Part print with two shaded views. Sizes in mm from the minimum x, y, z corner. A direction names the side the tool comes from. Round coordinates to 2 decimals unless told otherwise and drop trailing zeros. Order: outer loops, then holes, each group sorted by start corner. A loop starts at its lowest first (then second) coordinate and runs counter-clockwise, first axis right, second up. Notation, with made-up numbers: (27, 73.25) -> (44, 73.25) arc R32 cw to (44, 104.25) -> close; hole circle Ø3 at (-37.75, 48.5). An arc over 180 degrees is marked (long way). Use a Markdown table: item, result. Add a question column.
Item 1: 3-axis set-ups, long thin cutter, end or side, ignore diameter. For the marked faces 1 and 2: which of +Z, -Z, +X, -X, +Y, -Y reach the whole face in a straight line?
Item 2: Probe L1, parallel to Z at x = 8.75, y = 10; L2, parallel to Y at x = 6, z = 0.25; L3, parallel to X at y = 6.75, z = 0.25. List the from-to ranges inside material, lowest first.
Item 3: Slice it at D-D, the plane x = 8.25. Give the cut face in (y, z).
Item 4: Slice it at A-A, the plane x = 6. Give the cut face in (y, z), plus the area to 3 significant figures.
Item 5: Pin check, flat tips, straight feed: pin 1 (3.5 mm diameter, centred on x = 4, y = 7.5, fed in from +Z); pin 2 (0.5 mm diameter, centred on y = 12, z = 1.5, fed in from +X); pin 3 (2 mm diameter, centred on x = 5, y = 5, fed in from +Z); pin 4 (0.8 mm diameter, centred on y = 12, z = 1.5, fed in from -X). Stop position of each tip, or through.
Item 6: Slice it at B-B, the plane y = 6. Give the cut face in (x, z), plus the area to 3 significant figures.
Item 7: Slice it at C-C, the plane z = 0.35. Give the cut face in (x, y).
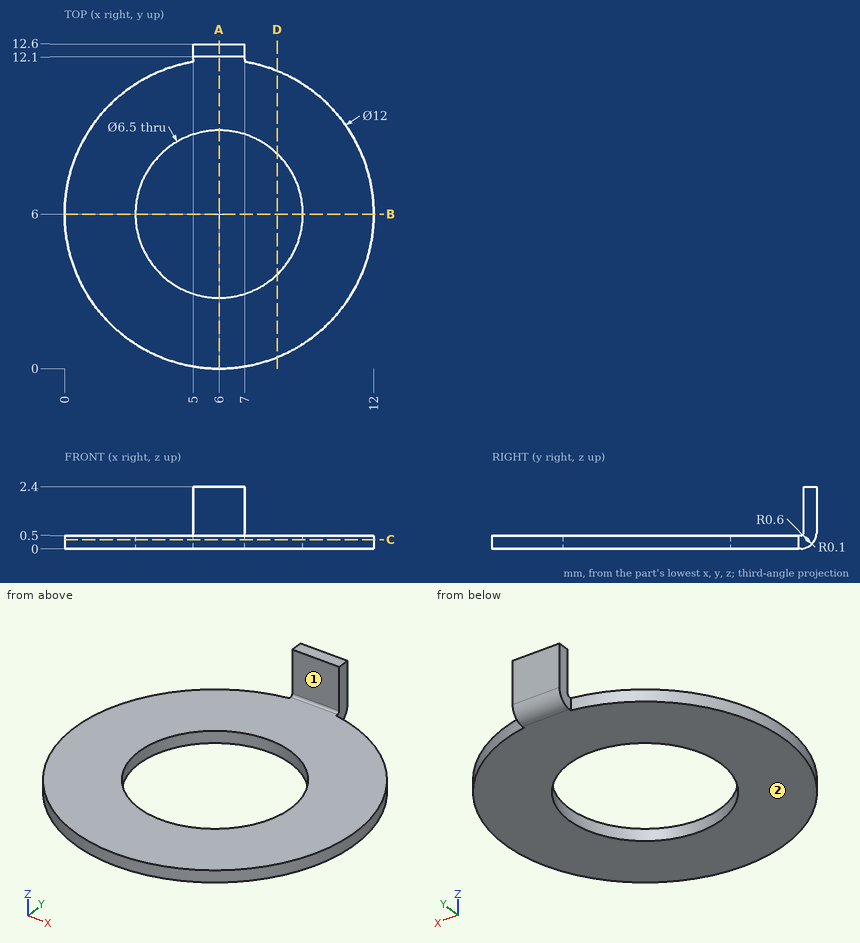
Check sheet entries:
| question | item | result |
|---|---|---|
| 1 | face 1 | +Z, +X, -X, -Y |
| 1 | face 2 | -Z, +X, -X, +Y, -Y |
| 2 | L1 | 0 to 0.5 |
| 2 | L2 | 0 to 2.75, 9.25 to 12.49 |
| 2 | L3 | 0.05 to 2.84, 9.16 to 11.95 |
| 3 | outline | (0.44, 0) -> (3.65, 0) -> (3.65, 0.5) -> (0.44, 0.5) -> close; (8.35, 0) -> (11.56, 0) -> (11.56, 0.5) -> (8.35, 0.5) -> close |
| 4 | outline | (0, 0) -> (2.75, 0) -> (2.75, 0.5) -> (0, 0.5) -> close; (9.25, 0) -> (12, 0) arc R0.6 ccw to (12.6, 0.6) -> (12.6, 2.4) -> (12.1, 2.4) -> (12.1, 0.6) arc R0.1 cw to (12, 0.5) -> (9.25, 0.5) -> close |
| 4 | area | 3.92 mm2 |
| 5 | pin 1 | z = 0.5 |
| 5 | pin 2 | x = 7 |
| 5 | pin 3 | through |
| 5 | pin 4 | x = 5 |
| 6 | outline | (0, 0) -> (2.75, 0) -> (2.75, 0.5) -> (0, 0.5) -> close; (9.25, 0) -> (12, 0) -> (12, 0.5) -> (9.25, 0.5) -> close |
| 6 | area | 2.75 mm2 |
| 7 | outline | (5, 11.92) arc R6 ccw (long way) to (7, 11.92) -> (7, 12.55) -> (5, 12.55) -> close; hole circle Ø6.5 at (6, 6) |
